Verification items for the finished model (mm, model axes). A direction names the side the tool comes from. Round coordinates to 2 decimals unless told otherwise and drop trailing zeros. Order: outer loops, then holes, each group sorted by start corner. A loop starts at its lowest first (then second) coordinate and runs counter-clockwise, first axis right, second up. Notation, with made-up numbers: M 32.25,37.5 L 36.25,37.5 A21 cw 36.25,49.5 Z; hole C 29,-17.5 d11. An arc over 180 degrees is marked long. Answer as a JSON object with one key per item and string values. Group by question number.
```python
from build123d import *

# Parameters (mm, degrees)
F0_R      = 40
F0_R_2    = 11.15
F1_DEPTH  = 7
F3_W      = 4.2920620181
F3_H      = 25.3791473806
F4_DEPTH  = 50
F5_W      = 38.4419448674
F5_H      = 3.5456162877
F6_DEPTH  = 25
F8_W      = 29.4845998287
F8_H      = 3.5456162877
F9_DEPTH  = 25
F12_R     = 1
F13_DEPTH = 6
F10_R     = 5.7969793016
F10_R_2   = 5.8597151437
F11_R     = 5.5483568343
F11_R_2   = 5.5921159978
F14_DEPTH = 6


with BuildPart() as f1:
    # F0 (on Top) → F1 (new body)
    with BuildSketch(Plane.XY):
        Circle(F0_R)
        Circle(F0_R_2, mode=Mode.SUBTRACT)
    extrude(amount=F1_DEPTH)

    # F3 (on face) → F4 (cut)
    with BuildSketch(Plane.XY.offset(7)):
        with Locations((0, 29.5779034495)):
            Rectangle(F3_W, F3_H)
    extrude(amount=-F4_DEPTH, mode=Mode.SUBTRACT)

    # F5 (on face) → F6 (cut)
    with BuildSketch(Plane.XY.offset(7)):
        with Locations((-35.5494692922, 0)):
            Rectangle(F5_W, F5_H)
    extrude(amount=-F6_DEPTH, mode=Mode.SUBTRACT)

    # F8 (on face) → F9 (cut)
    with BuildSketch(Plane.XY.offset(7)):
        with Locations((32.1904607117, 0)):
            Rectangle(F8_W, F8_H)
    extrude(amount=-F9_DEPTH, mode=Mode.SUBTRACT)

    # F12
    f12_edges = [f1.edges().sort_by_distance(p)[0] for p in [
        (-28.416076, 28.15185, 7),
        (-28.416076, 28.15185, 0),
        (0, -40, 0),
        (28.416076, 28.15185, 0),
        (0, -40, 7),
        (28.416076, 28.15185, 7),
    ]]
    fillet(f12_edges, radius=F12_R)

    # F7 (on face) → F13 (cut)
    with BuildSketch(Plane.XY.offset(7)):
        with BuildLine():
            ThreePointArc((-2.3326422088, -39.9319268296), (0, -40), (2.3326422088, -39.9319268296))
            Line((2.3326422088, -39.9319268296), (2.3326422088, -16.5151059628))
            Line((2.3326422088, -16.5151059628), (-2.3326422088, -16.5151059628))
            Line((-2.3326422088, -16.5151059628), (-2.3326422088, -39.9319268296))
        make_face()
    extrude(amount=-F13_DEPTH, mode=Mode.SUBTRACT)

    # F10 (on face) + F11 (on face) → F14 (cut)
    with BuildSketch(Plane.XY.offset(7)):
        with Locations((-20.6205584109, 20.6205565482)):
            Circle(F10_R)
        with Locations((-19.687499851, -17.4481645226)):
            Circle(F10_R_2)
    with BuildSketch(Plane.XY.offset(7)):
        with Locations((18.0079955608, 18.7544431537)):
            Circle(F11_R)
        with Locations((17.4481645226, -18.9410559833)):
            Circle(F11_R_2)
    extrude(amount=-F14_DEPTH, mode=Mode.SUBTRACT)


solid = f1.part
```
Q1. Tool access check on faces 1 (the face through (17, -19, 1)), 2 (the face through (17.448, 0, 4)), 3 (the face through (0, -16.515, 4)), 4 (the face through (-16.328, 0, 4)). Record the directions out of +Z, -Z, +X, -X, +Y, -Y that give a thin tool (end or side, any length) a straight path to the whole face; none if there is none.
Q2. Cross-section at B-B, the plane y = 0. Record the cut outline in (x, z), then the cut area to 3 significant figures.
Q3. Thickness scan on line 1 (Y direction, x = 0, z = 4.5); line 2 (Y direction, x = -25, z = 5.5); line 3 (X direction, y = -21.5, z = 1.5). Record the ranges inside material, lowest first. Write a range as from..to.
Q4. Release check for a two-part mould opening along X. For faces 5 (the face through (29, 1.773, 4)), 6 (the face through (-20, -17, 1)), 7 (the face through (-28.77, -27.79, 3.46)) record: released by +X, released by -X, zero draft, split by the parting line, or undercut.
Q5. Cross-section at A-A, the plane x = 0. Record the cut outline in (y, z).
Q6. Cross-section at C-C, the plane z = 3. Record the cut outline in (x, y), then the cut area to 3 significant figures.
Q7. Gauge pin test, flat ends, axial feed: pin 1 Ø3.5 at (x, z) = (0.5, 4) entering from -Y; pin 2 Ø3.5 at (x, y) = (-19.5, -19.5) entering from +Z; pin 3 Ø1 at (x, z) = (11.5, 4.5) entering from -Y. Record the tip position at first contact, or that the pin passes through.
Conclusion:
{
 "1": {"face 1": "+Z", "face 2": "+Z, -Z, +X", "face 3": "+Z, -Y", "face 4": "+Z, -Z, -X"},
 "2": {"outline": "M -16.33,0 L -11.15,0 L -11.15,7 L -16.33,7 Z; M 11.15,0 L 17.45,0 L 17.45,7 L 11.15,7 Z", "area": "80.3 mm2"},
 "3": {"line 1": "-16.52..-11.15, 11.15..16.89", "line 2": "-31.22..-19.92, -14.98..-1.77, 1.77..16.82, 24.42..31.22", "line 3": "-33.73..-23.92, -15.45..-2.33, 2.33..12.48, 22.42..33.73"},
 "4": {"face 5": "zero draft", "face 6": "undercut", "face 7": "released by -X"},
 "5": {"outline": "M -40,1 A1 ccw -39,0 L -11.15,0 L -11.15,7 L -16.52,7 L -16.52,1 Z; M 11.15,0 L 16.89,0 L 16.89,7 L 11.15,7 Z"},
 "6": {"outline": "M -39.96,-1.77 A40 ccw -2.33,-39.93 L -2.33,-16.52 L 2.33,-16.52 L 2.33,-39.93 A40 ccw 39.96,-1.77 L 17.45,-1.77 L 17.45,1.77 L 39.96,1.77 A40 ccw 2.15,39.94 L 2.15,16.89 L -2.15,16.89 L -2.15,39.94 A40 ccw -39.96,1.77 L -16.33,1.77 L -16.33,-1.77 Z; hole C -20.62,20.62 d11.59; hole C -19.69,-17.45 d11.72; hole C 0,0 d22.3; hole C 17.45,-18.94 d11.18; hole C 18.01,18.75 d11.1", "area": "3,860 mm2"},
 "7": {"pin 1": "y = -16.52", "pin 2": "z = 1", "pin 3": "y = -38.46"}
}
